Read the model definition and answer for the solid it produces. Units are mm, in the model's axes. Face numbers are marked on the shaded views. A direction names the side the tool comes from. Coordinates: 2 decimals unless noted, no trailing zeros. Write each loop counter-clockwise with the first axis right and the second up, starting at its lowest first coordinate (ties: lowest second). Pieces come first, ordered by that corner, then holes.
1) The part is cut by section B-B (z = 5). Determine the outline of the cut face in (x, y).
2) The part is cut by section A-A (x = -24.2). Determine the outline of the cut face in (y, z), then the cut area to 3 significant figures.
3) The part is cut by section D-D (x = -10). Determine the outline of the cut face in (y, z), then the cut area to 3 significant figures.
4) Which of the six approach directions +Z, -Z, +X, -X, +Y, -Y give full straight-line access (tool end or side, diameter ignored) to the marked faces 1, 2 and 3?
5) The part is cut by section C-C (z = 0). Determine the outline of the cut face in (x, y), then the cut area to 3 significant figures.
6) Each of these flat-tipped pins is pushed along its axis until it touches: pin 1 Ø7.5 at (x, z) = (-23, 4) entering from -Y; pin 2 Ø5 at (x, z) = (24.2, 5) entering from +Y; pin 3 Ø5 at (y, z) = (17, 6.5) entering from +X. Where does it stop, or does it pass through?
7) Find the intervals of material crossed by line 1 (Z direction, x = -24.2, y = 1.9); line 2 (X direction, y = 2, z = -5); line 3 (Y direction, x = -17, z = 1.25), in increasing order.
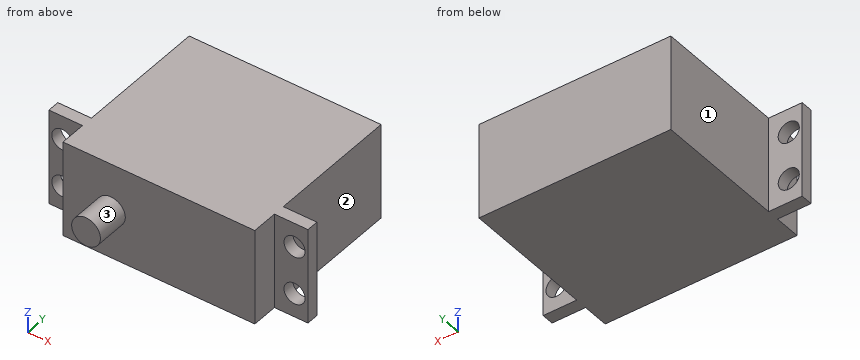
from build123d import *

# Parameters (mm, degrees)
SKETCH_1_W               = 40
SKETCH_1_H               = 20
EXTRUDE_2_DEPTH          = 30
SKETCH_3_W               = 54
SKETCH_3_H               = 20
EXTRUDE_3_DEPTH          = 2.5
CUT_EXTRUDE_3_DEPTH      = 42.581245773
CUT_EXTRUDE_3_DEPTH_BACK = 42.581245773
SKETCH_4_R               = 2.2
SKETCH_5_W               = 40
SKETCH_5_H               = 20
EXTRUDE_4_DEPTH          = 5.5
EXTRUDE_START            = -5.5
SKETCH_6_R               = 3
EXTRUDE_5_DEPTH          = 7


with BuildPart() as part:
    # 草图1 → 凸台-拉伸2 (new body)
    with BuildSketch(Plane(origin=(0, 0, 0), x_dir=(1, 0, 0), z_dir=(0, 1, 0))):
        Rectangle(SKETCH_1_W, SKETCH_1_H)
    extrude(amount=EXTRUDE_2_DEPTH)

    # 草图3 → 凸台-拉伸3 (add)
    with BuildSketch(Plane(origin=(0, 0, 0), x_dir=(1, 0, 0), z_dir=(0, 1, 0))):
        Rectangle(SKETCH_3_W, SKETCH_3_H)
    extrude(amount=EXTRUDE_3_DEPTH)

    # 草图4 → 切除-拉伸3 (cut, two sides: drawn at the far end of the back side and taken through both)
    with BuildSketch(Plane(origin=(0, 0, 0), x_dir=(1, 0, 0), z_dir=(0, 1, 0)).offset(-CUT_EXTRUDE_3_DEPTH_BACK)):
        with Locations(Location((-24.2, -5, 0), (0, 0, 270))):
            Circle(SKETCH_4_R)
        with Locations(Location((-24.2, 5, 0), (0, 0, 270))):
            Circle(SKETCH_4_R)
        with Locations(Location((24.2, -5, 0), (0, 0, 270))):
            Circle(SKETCH_4_R)
        with Locations(Location((24.2, 5, 0), (0, 0, 270))):
            Circle(SKETCH_4_R)
    extrude(amount=CUT_EXTRUDE_3_DEPTH + CUT_EXTRUDE_3_DEPTH_BACK, mode=Mode.SUBTRACT)

    # 草图5 → 凸台-拉伸4 (add)
    with BuildSketch(Plane(origin=(0, 0, 0), x_dir=(1, 0, 0), z_dir=(0, 1, 0))):
        Rectangle(SKETCH_5_W, SKETCH_5_H)
    extrude(amount=-EXTRUDE_4_DEPTH)

    # 草图6 → 凸台-拉伸5 (add)
    with BuildSketch(Plane(origin=(0, 0, 0), x_dir=(1, 0, 0), z_dir=(0, 1, 0)).offset(EXTRUDE_START)):
        with Locations(Location((-10, 0, 0), (0, 0, 90))):
            Circle(SKETCH_6_R)
    extrude(amount=-EXTRUDE_5_DEPTH)


solid = part.part
Reported:
1. outline: (-27, 0) - (-26.4, 0) - (-26.4, 2.5) - (-27, 2.5) - close; (-22, 0) - (-20, 0) - (-20, -5.5) - (20, -5.5) - (20, 0) - (22, 0) - (22, 2.5) - (20, 2.5) - (20, 30) - (-20, 30) - (-20, 2.5) - (-22, 2.5) - close; (26.4, 0) - (27, 0) - (27, 2.5) - (26.4, 2.5) - close
2. outline: (0, -10) - (2.5, -10) - (2.5, -7.2) - (0, -7.2) - close; (0, -2.8) - (2.5, -2.8) - (2.5, 2.8) - (0, 2.8) - close; (0, 7.2) - (2.5, 7.2) - (2.5, 10) - (0, 10) - close
2. area: 28.0 mm2
3. outline: (-12.5, -3) - (-5.5, -3) - (-5.5, -10) - (30, -10) - (30, 10) - (-5.5, 10) - (-5.5, 3) - (-12.5, 3) - close
3. area: 752 mm2
4. face 1: +Z, -Z, -X, +Y
4. face 2: +Z, -Z, +X, +Y
4. face 3: -Y
5. outline: (-27, 0) - (-20, 0) - (-20, -5.5) - (-13, -5.5) - (-13, -12.5) - (-7, -12.5) - (-7, -5.5) - (20, -5.5) - (20, 0) - (27, 0) - (27, 2.5) - (20, 2.5) - (20, 30) - (-20, 30) - (-20, 2.5) - (-27, 2.5) - close
5. area: 1,500 mm2
6. pin 1: stops at y = -5.5
6. pin 2: stops at y = 2.5
6. pin 3: stops at x = 20
7. line 1: z = -10 to -7.2, -2.8 to 2.8, 7.2 to 10
7. line 2: x = -27 to -26.4, -22 to 22, 26.4 to 27
7. line 3: y = -5.5 to 30
